Input: part model. Units: mm. Frame: model coordinates. A direction names the side the tool comes from. Coordinates: 2 decimals unless noted, no trailing zeros. Loops run counter-clockwise (first coordinate to the right, second up) from the corner with the lowest first, then second, coordinate; pieces in that order, holes last. Notation, with made-up numbers: (-16.5, -13) -> (-7.5, -13) arc R24 ccw to (-7.5, 23) -> close; hole circle Ø4 at (-35, 70.25). An arc over 180 degrees is marked (long way). Answer as a JSON object with one key per item and string values.
from build123d import *

# Parameters (mm, degrees)
SKETCH_1_W   = 9.5
SKETCH_1_H   = 6
SKETCH_1_W_2 = 4.85
SKETCH_1_H_2 = 7


with BuildPart() as part:
    # Эскиз1 → Повернуть1 (revolve)
    with BuildSketch(Plane.XY, mode=Mode.PRIVATE) as revolve_1_sk:
        with Locations((4.75, 64)):
            Rectangle(SKETCH_1_W, SKETCH_1_H)
        Polygon((9.5, 61), (0, 61), (0, 0), (4.85, 0), (13, 0), (13, 24), (11.5, 24), (11.5, 49), (9.5, 49), align=None)
        with Locations((2.425, -3.5)):
            Rectangle(SKETCH_1_W_2, SKETCH_1_H_2)
    revolve(revolve_1_sk.sketch.rotate(Axis((0, 73.447142448, 0), (0, -1, 0)), 90), axis=Axis((0, 73.447142448, 0), (0, -1, 0)))


solid = part.part
1. Section query C-C (y = 43.5). Return loops of the section in (x, z).
Reply:
{"outline": "circle Ø23 at (0, 0)"}
2. Section query B-B (x = 0). Return loops of the section in (y, z).
Reply:
{"outline": "(-7, -4.85) -> (0, -4.85) -> (0, -13) -> (24, -13) -> (24, -11.5) -> (49, -11.5) -> (49, -9.5) -> (67, -9.5) -> (67, 9.5) -> (49, 9.5) -> (49, 11.5) -> (24, 11.5) -> (24, 13) -> (0, 13) -> (0, 4.85) -> (-7, 4.85) -> close"}
3. Pin query (flat end, axial travel): P1, Ø1.5, axis at y = 20, z = 1.5, coming from the -X side; P2, Ø3, axis at x = -4, z = 7.5, coming from the -Y side; P3, Ø10, axis at y = 7.5, z = 10, coming from the +X side. Return the tip coordinate at first contact, or that it passes through.
Reply:
{"P1": "stops at x = -12.98", "P2": "stops at y = 0", "P3": "stops at x = 12"}
4. Section query D-D (z = 7.5). Return loops of the section in (x, y).
Reply:
{"outline": "(-10.62, 0) -> (10.62, 0) -> (10.62, 24) -> (8.72, 24) -> (8.72, 49) -> (5.83, 49) -> (5.83, 67) -> (-5.83, 67) -> (-5.83, 49) -> (-8.72, 49) -> (-8.72, 24) -> (-10.62, 24) -> close"}
5. Access query for faces 1 (the face through (0, -7, 0)), 2 (the face through (0, 0, -6)), 3 (the face through (9.274, 58.126, -2.059)). Directions: +Z, -Z, +X, -X, +Y, -Y. A direction counts if a zero-diameter tool reaches every point of the face in a straight line with its end or side. Return the directions, or none.
Reply:
{"face 1": "+Z, -Z, +X, -X, -Y", "face 2": "-Y", "face 3": "+Y"}
6. Line query: line 1 along Y through (x, z) = (-7.5, 10); line 2 along Y through (x, z) = (1, -8); line 3 along X through (y, z) = (46, -2). Output: solid intervals per line, ascending.
Reply:
{"line 1": "y = 0 to 24", "line 2": "y = 0 to 67", "line 3": "x = -11.32 to 11.32"}
7. Section query A-A (z = 0). Return loops of the section in (x, y), plus the area to 3 significant figures.
Reply:
{"outline": "(-13, 0) -> (-4.85, 0) -> (-4.85, -7) -> (4.85, -7) -> (4.85, 0) -> (13, 0) -> (13, 24) -> (11.5, 24) -> (11.5, 49) -> (9.5, 49) -> (9.5, 67) -> (-9.5, 67) -> (-9.5, 49) -> (-11.5, 49) -> (-11.5, 24) -> (-13, 24) -> close", "area": "1,610 mm2"}
